```python
from build123d import *

# Parameters (mm, degrees)
SKETCH1_R           = 4
BOSS_EXTRUDE1_DEPTH = 12
FILLET1_R           = 10


with BuildPart() as part:
    # Sketch1 → Boss-Extrude1 (new body)
    with BuildSketch(Plane.XY):
        with BuildLine():
            Line((333.691896068, 6), (6.708203932, 6))
            ThreePointArc((6.708203932, 6), (-9, 0), (6.708203932, -6))
            Line((6.708203932, -6), (333.691896068, -6))
            ThreePointArc((333.691896068, -6), (349.4001, 0), (333.691896068, 6))
        make_face()
        Circle(SKETCH1_R, mode=Mode.SUBTRACT)
        with Locations((340.4001, 0)):
            Circle(SKETCH1_R, mode=Mode.SUBTRACT)
    extrude(amount=BOSS_EXTRUDE1_DEPTH)

    # Fillet1
    fillet1_edges = [part.edges().sort_by_distance(p)[0] for p in [
        (6.708203932, 6, 6),
        (333.691896068, 6, 6),
        (333.691896068, -6, 6),
        (6.708203932, -6, 6),
    ]]
    fillet(fillet1_edges, radius=FILLET1_R)


solid = part.part
```
Input: part model. Units: mm. Frame: model coordinates. A direction names the side the tool comes from. Give positions to 0.01 mm unless a question says otherwise; leave off trailing zeros. Order: outer loops, then holes, each group sorted by start corner. A loop starts at its lowest first (then second) coordinate and runs counter-clockwise, first axis right, second up. Notation, with made-up numbers: (72.5, 50.25) - (91.5, 50.25) arc R18 cw to (91.5, 74.25) - close; hole circle Ø1 at (-11.5, 49.5). An arc over 180 degrees is marked (long way). One line per item, written item: value.
1. Line query: probe 1 along Y at (x, z) = (245.5, 2.5); probe 2 along X at (y, z) = (-7.75, 8.75); probe 3 along X at (y, z) = (7.25, 11.25). Output: solid intervals per line, ascending.
Determined:
probe 1: -6 to 6
probe 2: -4.58 to 4.58, 335.82 to 344.98
probe 3: -5.33 to 5.41, 334.99 to 345.73
2. Pin query (flat end, axial travel): pin 1 Ø1 at (y, z) = (-5, 7) entering from +X; pin 2 Ø1 at (y, z) = (-1, 5.5) entering from -X; pin 3 Ø1 at (x, z) = (96, 9.5) entering from -Y; pin 4 Ø5 at (x, y) = (340.4, 0) entering from -Z. Return the tip coordinate at first contact, or that it passes through.
Determined:
pin 1: x = 348.19
pin 2: x = -8.99
pin 3: y = -6
pin 4: through
3. Cut plane D-D, the plane x = 62. Output: boundary loops of the cut face in (y, z).
Determined:
outline: (-6, 0) - (6, 0) - (6, 12) - (-6, 12) - close
4. Cut plane B-B, the plane z = 6.5. Output: boundary loops of the cut face in (x, y).
Determined:
outline: (4.85, -7.58) arc R10 cw to (10.25, -6) - (330.15, -6) arc R10 cw to (335.55, -7.58) arc R9 ccw (long way) to (335.55, 7.58) arc R10 cw to (330.15, 6) - (10.25, 6) arc R10 cw to (4.85, 7.58) arc R9 ccw (long way) to start; hole circle Ø8 at (0, 0); hole circle Ø8 at (340.4, 0)
5. Cut plane A-A, the plane y = 0. Output: boundary loops of the cut face in (x, z), and give its area (3 significant figures).
Determined:
outline: (-9, 0) - (-4, 0) - (-4, 12) - (-9, 12) - close; (4, 0) - (336.4, 0) - (336.4, 12) - (4, 12) - close; (344.4, 0) - (349.4, 0) - (349.4, 12) - (344.4, 12) - close
area: 4,110 mm2
6. Reachability of faces 1 (the face through (332.92, 6.39, 6.08)), 2 (the face through (7.399, -6.414, 6.084)), 3 (the face through (349.396, -0.27, 5.916)) from +Z, -Z, +X, -X, +Y, -Y: full face, straight path, thin tool, end or side. Return the list, or none.
Determined:
face 1: +Z, -Z, +Y
face 2: +Z, -Z, -Y
face 3: +Z, -Z
7. Draft query along X for faces 4 (the face through (172, 6, 6)), 5 (the face through (168, 0, 12)). Return one class per face: released by +X, released by -X, zero draft, split by the parting line, or undercut.
Determined:
face 4: undercut
face 5: zero draft
8. Cut plane C-C, the plane x = 0. Output: boundary loops of the cut face in (y, z), and give its area (3 significant figures).
Determined:
outline: (-9, 0) - (-4, 0) - (-4, 12) - (-9, 12) - close; (4, 0) - (9, 0) - (9, 12) - (4, 12) - close
area: 120 mm2
